Answer from the drawing. Dimensions are ordinates in mm from the lowest x, y and z of the part. A direction names the side the tool comes from. Coordinates: 2 decimals unless noted, no trailing zeros. Order: outer loops, then holes, each group sorted by start corner. A loop starts at its lowest first (then second) coordinate and runs counter-clockwise, first axis right, second up. Notation, with made-up numbers: (-17.5, 39.25) -> (21.5, 39.25) arc R23 ccw to (21.5, 47.25) -> close; hole circle Ø1 at (42.25, 71.25). An arc over 180 degrees is marked (long way). Answer as a JSON object with one key per item and string values. Group by question number.
1) Section C-C on z = 3.5 is taken. Count the separate pieces of the cut face and the enclosed holes in it, and give its area (3 significant figures).
2) Consider L1, parallel to Y at x = 6.35, z = 1.8 (1 decimal); L2, parallel to X at y = 45, z = 2.75 (1 decimal); L3, parallel to Y at x = 44.5, z = 7. Determine where each line is inside the solid, lowest interval first.
3) Section A-A on x = 30 is taken. Determine the outline of the cut face in (y, z) (1 decimal).
4) Given pin 1 (2 mm diameter, centred on y = 42.5, z = 3, fed in from +X); pin 2 (5.5 mm diameter, centred on x = 57.11, y = 7.32, fed in from +Z) (3 decimals); pin 3 (2.5 mm diameter, centred on x = 63.5, z = 6, fed in from -Y); pin 4 (3 mm diameter, centred on x = 57.11, y = 7.32, fed in from +Z), each flat-ended and moving along its own axis, determine where each tip first touches the part or whether it passes through.
5) A tool of negligible diameter and unlimited length cuts with its end or side. For the marked faces 4 and 5, from which of +Z, -Z, +X, -X, +Y, -Y can it reach the whole face along a straight path? Write none if from no direction.
6) Determine the mould class of the marked faces 1, 2 and 3 for opening direction Y: released by +Y, released by -Y, zero draft, split by the parting line, or undercut.
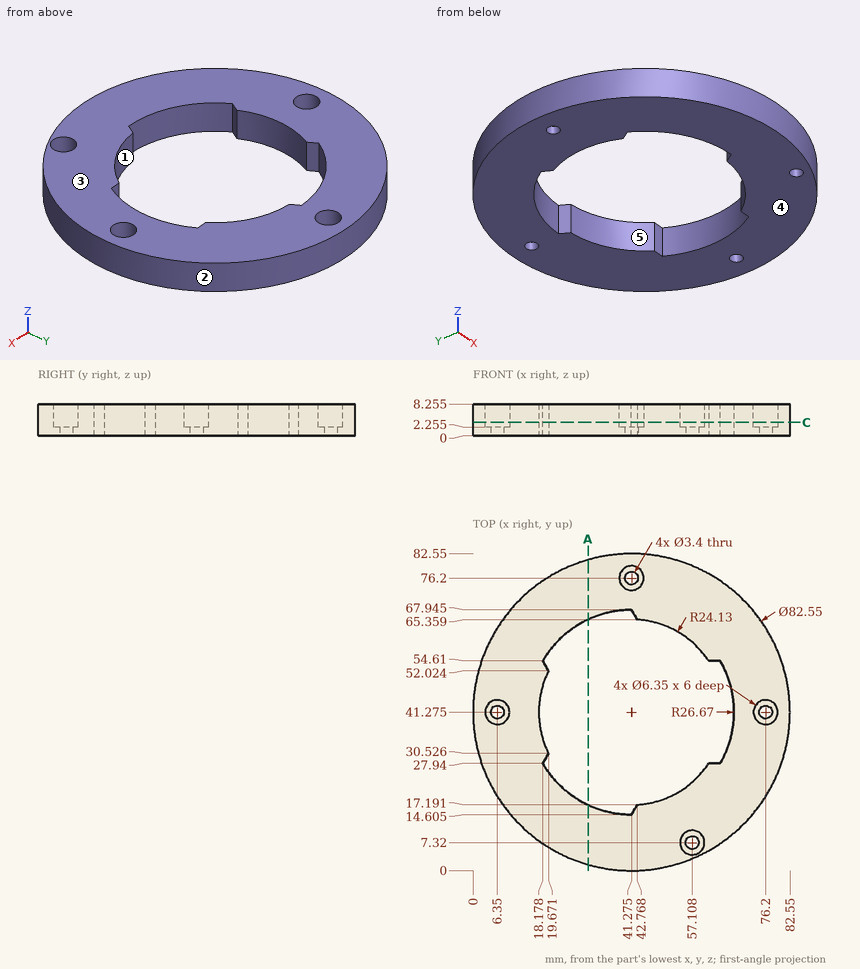
Worked answers:
{
 "1": {"separate pieces": "1", "enclosed holes": "5", "area": "3,180 mm²"},
 "2": {"L1": "y = 19.3 to 39.6, 43 to 63.3", "L2": "x = 0.2 to 17.4, 67.7 to 82.4", "L3": "y = 0.13 to 17.36, 65.19 to 82.42"},
 "3": {"outline": "(1.6, 0) -> (17.1, 0) -> (17.1, 8.3) -> (1.6, 8.3) -> close; (65.4, 0) -> (81, 0) -> (81, 8.3) -> (65.4, 8.3) -> close"},
 "4": {"pin 1": "stops at x = 82.55", "pin 2": "stops at z = 2.255", "pin 3": "stops at y = 5.73", "pin 4": "passes through"},
 "5": {"face 4": "-Z, +X, -X, +Y, -Y", "face 5": "+Z, -Z"},
 "6": {"face 1": "undercut", "face 2": "split by the parting line", "face 3": "zero draft"}
}
